from build123d import *

# Parameters (mm, degrees)
SKETCH2_R           = 12.7
SKETCH2_R_2         = 3.175
BOSS_EXTRUDE1_DEPTH = 5
SKETCH3_R           = 6
SKETCH3_R_2         = 3.175
BOSS_EXTRUDE2_DEPTH = 4.2
CUT_EXTRUDE1_REACH  = 20.643
SKETCH4_R           = 1.1303
CIRPATTERN1_COUNT   = 6


with BuildPart() as part:
    # Sketch2 → Boss-Extrude1 (new body)
    with BuildSketch(Plane.XY):
        Circle(SKETCH2_R)
        Circle(SKETCH2_R_2, mode=Mode.SUBTRACT)
    extrude(amount=BOSS_EXTRUDE1_DEPTH)

    # Sketch3 → Boss-Extrude2 (add)
    with BuildSketch(Plane.XY.offset(5)):
        Circle(SKETCH3_R)
        Circle(SKETCH3_R_2, mode=Mode.SUBTRACT)
    extrude(amount=BOSS_EXTRUDE2_DEPTH)

    # Sketch4 → Cut-Extrude1 (cut, up to next)
    with BuildSketch(Plane.XY.offset(5), mode=Mode.PRIVATE) as cut_extrude1_sk1:
        with Locations((0, 9.525)):
            Circle(SKETCH4_R)
    cut_extrude1_tool1 = extrude(cut_extrude1_sk1.sketch, amount=-CUT_EXTRUDE1_REACH, mode=Mode.PRIVATE) & part.part
    cut_extrude1 = cut_extrude1_tool1.solids().sort_by_distance((0, 9.525, 5))[0]
    add(cut_extrude1, mode=Mode.SUBTRACT)

    # CirPattern1: Cut-Extrude1 ×6 about axis
    cirpattern1_axis = Axis((0, 0, 0), (0, 0, 1))
    for i in range(1, CIRPATTERN1_COUNT):
        add(cut_extrude1.rotate(cirpattern1_axis, i * 360 / CIRPATTERN1_COUNT), mode=Mode.SUBTRACT)


solid = part.part
Here's how the part is built. I have some questions about the finished solid (model axes, mm). A direction names the side the tool comes from. Round coordinates to 2 decimals unless told otherwise and drop trailing zeros. Write each loop counter-clockwise with the first axis right and the second up, starting at its lowest first coordinate (ties: lowest second). Pieces come first, ordered by that corner, then holes.
1. Suppose I cut it at C-C (z = 4). State how many separate pieces and enclosed holes the cut face has, and give its area (3 significant figures).
2. Will these pins go through, and if not, where does the flat tip stop? pin 1 Ø4 at (x, z) = (6.5, 6.5) entering from +Y; pin 2 Ø2 at (x, y) = (0, -9.525) entering from +Z; pin 3 Ø4 at (y, z) = (9, 4) entering from +X; pin 4 Ø3.5 at (x, y) = (8.25, -4.76) entering from +Z.
3. For faces 1 (the cylindrical face through (7.205, 5.195, 2.535)), 2 (the cylindrical face through (-6, 0, 7)), which set-ups out of +Z, -Z, +X, -X, +Y, -Y let a thin tool reach every point of the face, with its end or its side?
4. Suppose I cut it at B-B (x = 0). List the corners of the cut face in (y, z) for me (3 decimals).
5. Suppose I cut it at A-A (y = 0). List the corners of the cut face in (x, z) for me (3 decimals).
6. If we mould it in two halves opening along Y, with no side actions, what happens to faces 3 (the flat face through (3, -3, 0)), 4 (the cylindrical face through (-2.75, -12.4, 2.46)), 5 (the cylindrical face through (-7.17, -4.42, 2.54))? For each: released by +Y, released by -Y, zero draft, split by the parting line, or undercut.
7. I need wall thicknesses on L1, parallel to Y at x = 0, z = 4.25 (3 decimals); L2, parallel to Y at x = -7.25, z = 3.5; L3, parallel to Z at x = -3.25, y = 6. Which ranges of each line are inside material? Lowest first, please.
8. Suppose I cut it at D-D (z = 8.5). List the corners of the cut face in (x, y) for me (3 decimals), and give its area (3 significant figures).
Answer sheet:
1. separate pieces: 1
1. enclosed holes: 7
1. area: 451 mm2
2. pin 1: stops at y = 11.6
2. pin 2: passes through
2. pin 3: stops at x = 10.6
2. pin 4: stops at z = 5
3. face 1: +Z, -Z
3. face 2: +Z
4. outline: (-12.7, 0) - (-10.655, 0) - (-10.655, 5) - (-12.7, 5) - close; (-8.395, 0) - (-3.175, 0) - (-3.175, 9.2) - (-6, 9.2) - (-6, 5) - (-8.395, 5) - close; (3.175, 0) - (8.395, 0) - (8.395, 5) - (6, 5) - (6, 9.2) - (3.175, 9.2) - close; (10.655, 0) - (12.7, 0) - (12.7, 5) - (10.655, 5) - close
5. outline: (-12.7, 0) - (-3.175, 0) - (-3.175, 9.2) - (-6, 9.2) - (-6, 5) - (-12.7, 5) - close; (3.175, 0) - (12.7, 0) - (12.7, 5) - (6, 5) - (6, 9.2) - (3.175, 9.2) - close
6. face 3: zero draft
6. face 4: split by the parting line
6. face 5: undercut
7. L1: y = -12.7 to -10.655, -8.395 to -3.175, 3.175 to 8.395, 10.655 to 12.7
7. L2: y = -10.43 to -5.29, -4.23 to 4.23, 5.29 to 10.43
7. L3: z = 0 to 5
8. outline: circle Ø12 at (0, 0); hole circle Ø6.35 at (0, 0)
8. area: 81.4 mm2
